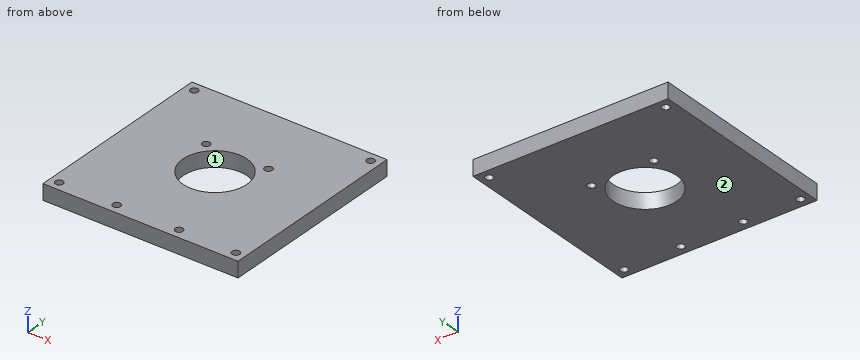
from build123d import *

# Parameters (mm, degrees)
SKETCH1_W           = 50
SKETCH1_H           = 50
SKETCH1_R           = 1
BOSS_EXTRUDE1_DEPTH = 4
SKETCH2_R           = 8.2
SKETCH2_R_2         = 1
CUT_EXTRUDE1_DEPTH  = 10


with BuildPart() as part:
    # Sketch1 → Boss-Extrude1 (new body)
    with BuildSketch(Plane.XY):
        Rectangle(SKETCH1_W, SKETCH1_H)
        with Locations((-22.627416998, 22.627416998)):
            Circle(SKETCH1_R, mode=Mode.SUBTRACT)
        with Locations((22.627416998, 22.627416998)):
            Circle(SKETCH1_R, mode=Mode.SUBTRACT)
        with Locations((22.627416998, -22.627416998)):
            Circle(SKETCH1_R, mode=Mode.SUBTRACT)
        with Locations((-22.627416998, -22.627416998)):
            Circle(SKETCH1_R, mode=Mode.SUBTRACT)
    extrude(amount=BOSS_EXTRUDE1_DEPTH)

    # Sketch2 → Cut-Extrude1 (cut)
    with BuildSketch(Plane.XY.offset(4)):
        Circle(SKETCH2_R)
        with Locations((-8, 7.5)):
            Circle(SKETCH2_R_2)
        with Locations((8, 7.5)):
            Circle(SKETCH2_R_2)
        with Locations((-8, -22.5)):
            Circle(SKETCH2_R_2)
        with Locations((8, -22.5)):
            Circle(SKETCH2_R_2)
    extrude(amount=-CUT_EXTRUDE1_DEPTH, mode=Mode.SUBTRACT)


solid = part.part
Design review of the part built by this model. Coordinates are the model's own, in mm. Face numbers are marked on the shaded views. Coordinates: 2 decimals unless noted, no trailing zeros. Order: outer loops, then holes, each group sorted by start corner. A loop starts at its lowest first (then second) coordinate and runs counter-clockwise, first axis right, second up.
Item 1: For line 1 (Y direction, x = 22.5, z = 0.25); line 2 (Y direction, x = -23, z = 2.6); line 3 (Y direction, x = -5.5, z = 1.5), list the stretches that pass through material, from the lowest coordinate up.
Item 2: For pin 1 Ø1.6 at (x, y) = (-8, -22.5) entering from -Z, flat-tipped, find the tip position at first contact; note if it passes through.
Item 3: Take a section at D-D, the plane x = 22.5. Write out the cut boundary in (y, z), then the cut area to 3 significant figures.
Item 4: The part is to be moulded in two halves that separate along Y. For the marked faces 1 and 2, say which applies: pulls with the +Y half, pulls with the -Y half, needs draft (parallel to the pull), parting line crosses it, or undercut.
Item 5: Take a section at C-C, the plane z = 2.55. Count the separate pieces of the cut face and the enclosed holes in it, then the cut area to 3 significant figures.
Item 6: Take a section at A-A, the plane y = 0. Write out the cut boundary in (x, z), then the cut area to 3 significant figures.
The answers:
1. line 1: y = -25 to -23.62, -21.64 to 21.64, 23.62 to 25
1. line 2: y = -25 to -23.56, -21.7 to 21.7, 23.56 to 25
1. line 3: y = -25 to -6.08, 6.08 to 25
2. pin 1: passes through
3. outline: (-25, 0) - (-23.62, 0) - (-23.62, 4) - (-25, 4) - close; (-21.64, 0) - (21.64, 0) - (21.64, 4) - (-21.64, 4) - close; (23.62, 0) - (25, 0) - (25, 4) - (23.62, 4) - close
3. area: 184 mm2
4. face 1: undercut
4. face 2: needs draft
5. separate pieces: 1
5. enclosed holes: 9
5. area: 2,260 mm2
6. outline: (-25, 0) - (-8.2, 0) - (-8.2, 4) - (-25, 4) - close; (8.2, 0) - (25, 0) - (25, 4) - (8.2, 4) - close
6. area: 134 mm2
